Geometry check sheet. Reference: drawing and pictorial views, mm from the part's lowest x, y, z. Give positions to 0.01 mm unless a question says otherwise; leave off trailing zeros. Order: outer loops, then holes, each group sorted by start corner. A loop starts at its lowest first (then second) coordinate and runs counter-clockwise, first axis right, second up. Notation, with made-up numbers: M 68,-14.5 L 104,-14.5 A8 ccw 104,-4.5 Z; hole C 56.25,3 d6. An arc over 180 degrees is marked long. Use CSV: the item, a comma, the result in double quotes. Start each with the question number.
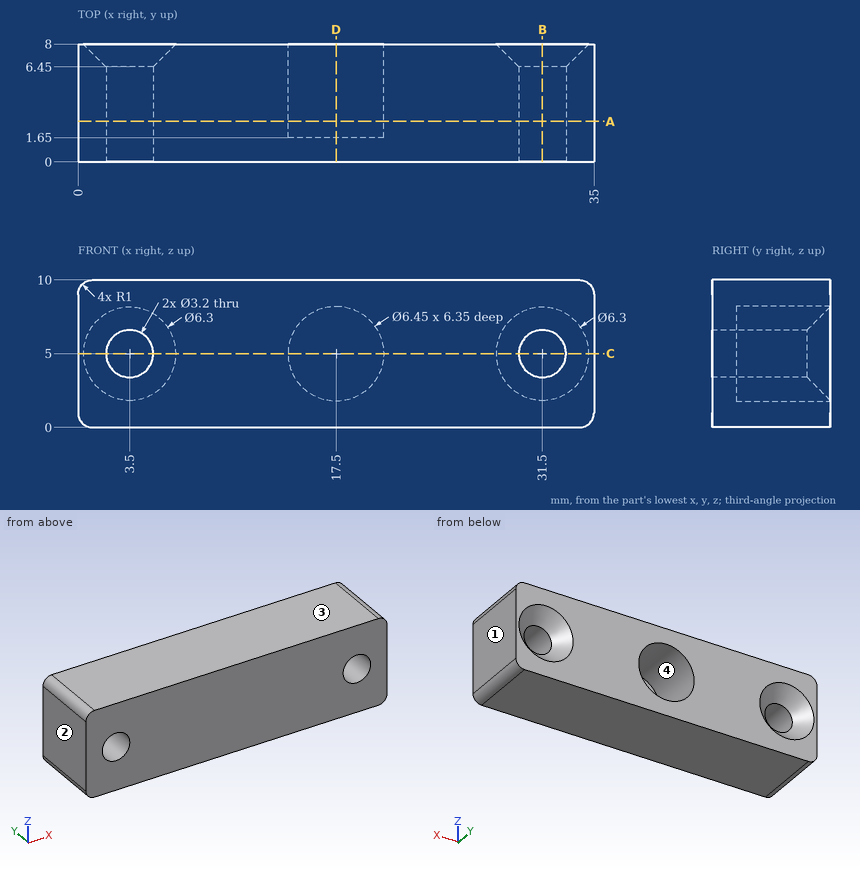
(1) Sectioned sample at A-A on y = 2.75. Record the cut outline in (x, z) (3 decimals), then the cut area to 3 significant figures.
(2) Go/stop test with a flat-tipped pin: P1, Ø3.5, axis at x = 31.5, z = 5, coming from the +Y side. Record where the tip stops, or that it passes through.
(3) Sectioned sample at B-B on x = 31.5. Record the cut outline in (y, z).
(4) Draft check along X on the marked faces 1, 2, 3 and 4. Enter one of: +X half, -X half, draft (parallel to the pull), parting line (faces both ways), or undercut.
(5) Sectioned sample at C-C on z = 5. Record the cut outline in (x, y) (3 decimals).
(6) Thickness scan on line 1 (X direction, y = 5.25, z = 5) (3 decimals); line 2 (Z direction, x = 3.5, y = 2.75); line 3 (X direction, y = 3.5, z = 4). Record the ranges inside material, lowest first.
(7) Sectioned sample at D-D on x = 17.5. Record the cut outline in (y, z) (3 decimals).
Responses:
1,outline,"M 0,1 A1 ccw 1,0 L 34,0 A1 ccw 35,1 L 35,9 A1 ccw 34,10 L 1,10 A1 ccw 0,9 Z; hole C 3.5,5 d3.2; hole C 17.5,5 d6.45; hole C 31.5,5 d3.2"
1,area,"300 mm2"
2,P1,"y = 6.6"
3,outline,"M 0,0 L 8,0 L 8,1.85 L 6.45,3.4 L 0,3.4 Z; M 0,6.6 L 6.45,6.6 L 8,8.15 L 8,10 L 0,10 Z"
4,face 1,"+X half"
4,face 2,"-X half"
4,face 3,"draft"
4,face 4,"undercut"
5,outline,"M 0,0 L 1.9,0 L 1.9,6.45 L 0.35,8 L 0,8 Z; M 5.1,0 L 29.9,0 L 29.9,6.45 L 28.35,8 L 20.725,8 L 20.725,1.65 L 14.275,1.65 L 14.275,8 L 6.65,8 L 5.1,6.45 Z; M 33.1,0 L 35,0 L 35,8 L 34.65,8 L 33.1,6.45 Z"
6,line 1,"0 to 1.9, 5.1 to 14.275, 20.725 to 29.9, 33.1 to 35"
6,line 2,"0 to 3.4, 6.6 to 10"
6,line 3,"0 to 2.25, 4.75 to 14.43, 20.57 to 30.25, 32.75 to 35"
7,outline,"M 0,0 L 8,0 L 8,1.775 L 1.65,1.775 L 1.65,8.225 L 8,8.225 L 8,10 L 0,10 Z"
